Autodesk Inventor part; units mm, degrees
ref_plane "YZ Plane" through (0, 0, 0) normal (1, 0, 0) x (0, 1, 0)
ref_plane "XZ Plane" through (0, 0, 0) normal (0, 1, 0) x (-1, 0, 0)
ref_plane "XY Plane" through (0, 0, 0) normal (0, 0, 1) x (1, 0, 0)
sketch "Sketch1" plane through (0, 0, 0) normal (0, 0, 1) x (1, 0, 0)
  line L0 (13.3295, 18.9186) -> (13.3295, 3.9186)
  line L1 (13.3295, 3.9186) -> (45.3295, 3.9186)
  line L2 (45.3295, 3.9186) -> (45.3295, 18.9186)
  line L3 (11.3295, 18.9186) -> (11.3295, 1.9186)
  line L4 (11.3295, 1.9186) -> (47.3295, 1.9186)
  line L5 (47.3295, 1.9186) -> (47.3295, 18.9186)
  line L6 (13.3295, 18.9186) -> (11.3295, 18.9186)
  line L7 (45.3295, 18.9186) -> (47.3295, 18.9186)
  point P0 (0, 0)
  dimension "d0" = 15
  dimension "d1" = 32
  dimension "d2" = 2
extrude "Extrusion1" add sketch "Sketch1" along normal blind 100
sketch "Sketch2" plane through (13.3295, 3.9186, 0) normal (0, 1, 0) x (1, 0, 0)
  line L0 (34, -100) -> (32, -100)
  line L1 (34, -100) -> (-2.138, -28.2724)
  line L2 (34, -100) -> (114.3169, -100) construction
  line L3 (32, -100) -> (0, -100)
  line L4 (34, -100) -> (-2.138, -100)
  line L5 (-2.138, -100) -> (-2.138, -28.2724)
  line L6 (-2.138, -28.2724) -> (15.4098, -63.1016)
  line L7 (15.4098, -63.1016) -> (34, -63.1016)
  line L8 (34, 0) -> (34, -100)
  point P0 (-13.3295, 0)
  point P1 (0, -100)
  dimension "d5" = 116.74
  dimension "d6" = 63.26
  dimension "d9" = 39
extrude "Extrusion2" cut sketch "Sketch2" along normal through all both and the other way through all
sketch "Sketch3" plane through (45.3295, 3.9186, 0) normal (-1, 0, 0) x (0, 0, 1)
  line L0 (63.1016, 0) -> (63.1016, 15)
  line L1 (63.1016, 15) -> (65.1016, 15)
  line L2 (65.1016, 15) -> (65.1016, -2)
  line L3 (65.1016, -2) -> (63.1016, -2)
  line L4 (63.1016, -2) -> (63.1016, 15)
  point P0 (0, -3.9186)
  dimension "d10" = 2
  dimension "d11" = 17
extrude "Extrusion3" add sketch "Sketch3" along normal blind 17 and the other way blind 2
properties part number "outside2"
Geometry check sheet. Reference: the model listing, model coordinates, mm. A direction names the side the tool comes from. Round coordinates to 2 decimals unless told otherwise and drop trailing zeros. Loops run counter-clockwise (first coordinate to the right, second up) from the corner with the lowest first, then second, coordinate; pieces in that order, holes last. Notation, with made-up numbers: (1.5, -5) - (32.5, -5) arc R25 ccw to (32.5, 20) - close; hole circle Ø4 at (4.25, -33). An arc over 180 degrees is marked (long way). Write each question's results on one line, items separated by ' | '. Start each with the question number.
Q1. Cross-section at A-A on y = 10.75. Enter the section's corners in (x, z), and give its area (3 significant figures).
Q2. Cross-section at B-B on z = 5.5. Enter the section's corners in (x, y).
Q3. Access from +Z, -Z, +X, -X, +Y, -Y to the whole of each face (thin tool, end or side, straight path). Record for faces 4 (the flat face through (29, 3.919, 31)), 5 (the flat face through (11.33, 11, 14)).
Q4. Cross-section at C-C on x = 41. Enter the section's corners in (y, z).
Q5. Thickness scan on line 1 (X direction, y = 7.5, z = 15); line 2 (Y direction, x = 33.5, z = 39.5); line 3 (X direction, y = 4.5, z = 38.5). Record the ranges inside material, lowest first. Write a range as [from, to].
Q6. Cross-section at D-D on z = 37.5. Enter the section's corners in (x, y), and give its area (3 significant figures).
Q7. Release check for a two-part mould opening along X. For faces 1 (the flat face through (47.33, 10, 32)), 2 (the flat face through (29, 1.919, 32)), 3 (the flat face through (13.33, 12, 16)) record: +X half, -X half, draft (parallel to the pull), parting line (faces both ways), or undercut.
Q8. Gauge pin test, flat ends, axial feed: P1, Ø1.5, axis at y = 9, z = 36, coming from the -X side; P2, Ø0.6, axis at y = 13, z = 64.5, coming from the -X side; P3, Ø3, axis at x = 37.5, z = 32, coming from the +Y side. Record the tip position at first contact, or that the pin passes through.
Answers below:
1) outline: (11.33, 0) - (13.33, 0) - (13.33, 32.52) - (11.33, 28.55) - close; (28.33, 63.1) - (45.33, 63.1) - (45.33, 0) - (47.33, 0) - (47.33, 65.1) - (28.33, 65.1) - close | area: 225 mm²
2) outline: (11.33, 1.92) - (47.33, 1.92) - (47.33, 18.92) - (45.33, 18.92) - (45.33, 3.92) - (13.33, 3.92) - (13.33, 18.92) - (11.33, 18.92) - close
3) face 4: -Z, +Y | face 5: +Z, -Z, -X, +Y, -Y
4) outline: (1.92, 0) - (3.92, 0) - (3.92, 63.1) - (18.92, 63.1) - (18.92, 65.1) - (1.92, 65.1) - close
5) line 1: x = [11.33, 13.33], [45.33, 47.33] | line 2: y = [1.92, 3.92] | line 3: x = [45.33, 47.33]
6) outline: (15.84, 1.92) - (47.33, 1.92) - (47.33, 18.92) - (45.33, 18.92) - (45.33, 3.92) - (15.84, 3.92) - close | area: 93.0 mm²
7) face 1: +X half | face 2: draft | face 3: undercut
8) P1: stops at x = 45.33 | P2: stops at x = 28.33 | P3: stops at y = 3.92
